```python
from build123d import *

# Parameters (mm, degrees)
F1_DEPTH = 6.5
F2_DEPTH = 2
F3_R     = 0.95
F4_DEPTH = 25
F5_R     = 2
F6_R     = 2


with BuildPart() as f1:
    # F0 (on Front) → F1 (new body)
    with BuildSketch(Plane.XZ):
        with BuildLine():
            Line((4.29925, -14.837718), (4.29925, -5.837718))
            ThreePointArc((4.29925, -5.837718), (0, 7.25), (-4.29925, -5.837718))
            Line((-4.29925, -5.837718), (-4.29925, -14.837718))
            Line((-4.29925, -14.837718), (-0.29925, -14.837718))
            Line((-0.29925, -14.837718), (-0.29925, -5.241464))
            ThreePointArc((-0.29925, -5.241464), (0, 5.25), (0.29925, -5.241464))
            Line((0.29925, -5.241464), (0.29925, -14.837718))
            Line((0.29925, -14.837718), (4.29925, -14.837718))
        make_face()
    extrude(amount=F1_DEPTH)

    # F0 (on Front) → F2 (join)
    with BuildSketch(Plane.XZ):
        with BuildLine():
            Line((0.29925, -3.738041), (0.29925, -5.241464))
            ThreePointArc((0.29925, -5.241464), (0, 5.25), (-0.29925, -5.241464))
            Line((-0.29925, -5.241464), (-0.29925, -3.738041))
            ThreePointArc((-0.29925, -3.738041), (0, 3.75), (0.29925, -3.738041))
        make_face()
    extrude(amount=F2_DEPTH)

    # F3 (on face) → F4 (cut)
    with BuildSketch(Plane.YZ.offset(4.29925)):
        with Locations((-3.25, -12.637718)):
            Circle(F3_R)
    extrude(amount=-F4_DEPTH, mode=Mode.SUBTRACT)

    # F5
    f5_edges = [f1.edges().sort_by_distance(p)[0] for p in [
        (2.29925, 0, -14.837718),
        (-2.29925, 0, -14.837718),
        (2.29925, -6.5, -14.837718),
        (-2.29925, -6.5, -14.837718),
    ]]
    fillet(f5_edges, radius=F5_R)

    # F6
    f6_edges = [f1.edges().sort_by_distance(p)[0] for p in [
        (4.29925, -3.25, -5.837718),
        (-4.29925, -3.25, -5.837718),
    ]]
    fillet(f6_edges, radius=F6_R)


solid = f1.part
```
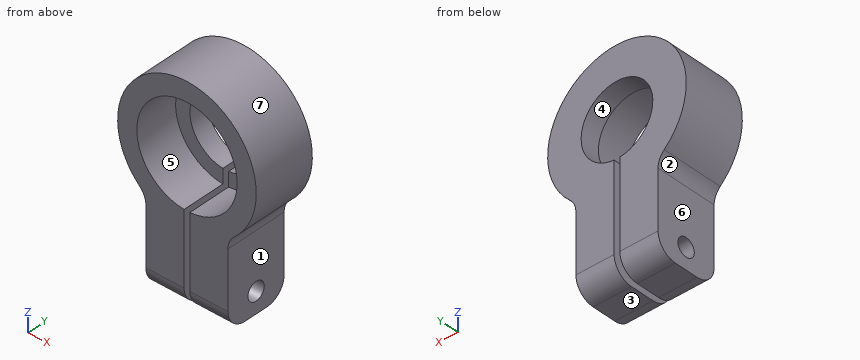
Design review of the part built by this model. Coordinates are the model's own, in mm. Face numbers are marked on the shaded views. A direction names the side the tool comes from. Round coordinates to 2 decimals unless told otherwise and drop trailing zeros. Write each loop counter-clockwise with the first axis right and the second up, starting at its lowest first coordinate (ties: lowest second). Pieces come first, ordered by that corner, then holes.
Item 1: We need section B-B on y = -3.25. Write out the cut boundary in (x, z).
Item 2: For the marked faces 5, 6 and 7, list the 3-axis set-ups (+Z, -Z, +X, -X, +Y, -Y) from which the entire face can be reached by the end or side of a thin tool; tool diameter is ignored.
Item 3: We need section D-D on x = -1. Write out the cut boundary in (y, z).
Item 4: We need section C-C on x = 2. Write out the cut boundary in (y, z).
Item 5: Clearance check with flat-ended pins moving along their axes: pin 1 Ø1.5 at (x, y) = (1.5, -2.5) entering from +Z; pin 2 Ø3 at (y, z) = (-2, -12) entering from -X; pin 3 Ø1.5 at (y, z) = (-3, -6) entering from +X. State where each tip first meets the part, or that it passes through.
Item 6: For probe 1 along X at (y, z) = (-3.5, -10); probe 2 along X at (y, z) = (-1.1, 0); probe 3 along Z at (x, y) = (-2.9, -3.25), list the stretches that pass through material, from the lowest coordinate up.
Item 7: The part is to be moulded in two halves that separate along X. For the marked faces 1, 2, 3 and 4, say which applies: +X half, -X half, draft (parallel to the pull), parting line (faces both ways), or undercut.
Item 8: We need section A-A on z = 0. Write out the cut boundary in (x, y).
Returned:
1. outline: (-4.94, -5.31) arc R2 cw to (-4.3, -6.77) - (-4.3, -11.69) - (-0.3, -11.69) - (-0.3, -5.24) arc R5.25 cw (long way) to (0.3, -5.24) - (0.3, -11.69) - (4.3, -11.69) - (4.3, -6.77) arc R2 cw to (4.94, -5.31) arc R7.25 ccw (long way) to start; (-4.3, -14.84) - (-0.3, -14.84) - (-0.3, -13.59) - (-4.3, -13.59) - close; (0.3, -14.84) - (4.3, -14.84) - (4.3, -13.59) - (0.3, -13.59) - close
2. face 5: -Y
2. face 6: -Z, -X, +Y, -Y
2. face 7: +Y, -Y
3. outline: (-6.5, -12.84) arc R2 ccw to (-4.5, -14.84) - (-2, -14.84) arc R2 ccw to (0, -12.84) - (0, -3.61) - (-2, -3.61) - (-2, -5.15) - (-6.5, -5.15) - close; (-6.5, 5.15) - (-2, 5.15) - (-2, 3.61) - (0, 3.61) - (0, 7.18) - (-6.5, 7.18) - close; hole circle Ø1.9 at (-3.25, -12.64)
4. outline: (-6.5, -12.84) arc R2 ccw to (-4.5, -14.84) - (-2, -14.84) arc R2 ccw to (0, -12.84) - (0, -3.17) - (-2, -3.17) - (-2, -4.85) - (-6.5, -4.85) - close; (-6.5, 4.85) - (-2, 4.85) - (-2, 3.17) - (0, 3.17) - (0, 6.97) - (-6.5, 6.97) - close; hole circle Ø1.9 at (-3.25, -12.64)
5. pin 1: stops at z = 7.21
5. pin 2: stops at x = -4.3
5. pin 3: stops at x = 5
6. probe 1: x = -4.3 to -0.3, 0.3 to 4.3
6. probe 2: x = -7.25 to -3.75, 3.75 to 7.25
6. probe 3: z = -14.84 to -13.59, -11.69 to -4.38, 4.38 to 6.64
7. face 1: +X half
7. face 2: -X half
7. face 3: draft
7. face 4: undercut
8. outline: (-7.25, -6.5) - (-5.25, -6.5) - (-5.25, -2) - (-3.75, -2) - (-3.75, 0) - (-7.25, 0) - close; (3.75, -2) - (5.25, -2) - (5.25, -6.5) - (7.25, -6.5) - (7.25, 0) - (3.75, 0) - close
